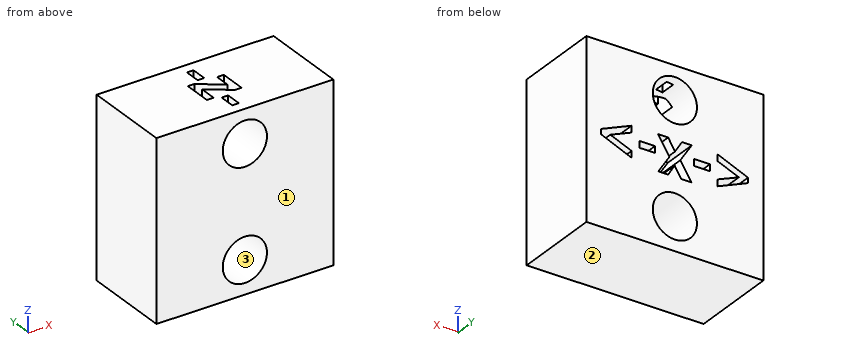
Autodesk Inventor part; units mm, degrees
ref_plane "YZ Plane" through (0, 0, 0) normal (1, 0, 0) x (0, 1, 0)
ref_plane "XZ Plane" through (0, 0, 0) normal (0, 1, 0) x (-1, 0, 0)
ref_plane "XY Plane" through (0, 0, 0) normal (0, 0, 1) x (1, 0, 0)
sketch "Sketch1" plane through (0, 0, 0) normal (0, 1, 0) x (-1, 0, 0)
  line L0 (12.7, 12.7) -> (-12.7, 12.7)
  line L1 (-12.7, 12.7) -> (-12.7, -12.7)
  line L2 (-12.7, -12.7) -> (12.7, -12.7)
  line L3 (12.7, -12.7) -> (12.7, 12.7)
  line L4 (12.7, 12.7) -> (-12.7, -12.7) construction
  line L5 (-12.7, 12.7) -> (12.7, -12.7) construction
  point P0 (0, 0)
  dimension "d0" = 25.4
  dimension "d1" = 25.4
extrude "Extrusion1" add sketch "Sketch1" along normal blind 12.7
sketch "Sketch2" plane through (0, 12.7, 0) normal (0, 1, 0) x (1, 0, 0)
  line L0 (-12.7, 12.7) -> (-12.7, -12.7) construction
  line L1 (-12.7, 0) -> (12.7, 0) construction
  line L2 (12.7, -12.7) -> (12.7, 12.7) construction
  line L3 (-6.1256, -2.4906) -> (-10.5058, -0.671)
  line L4 (-10.5058, -0.671) -> (-10.5058, 0.0782)
  line L5 (-10.5058, 0.0782) -> (-6.1256, 1.8978)
  line L6 (-6.1256, 1.8978) -> (-6.1256, 0.9551)
  line L7 (-6.1256, 0.9551) -> (-9.1885, -0.3005)
  line L8 (-9.1885, -0.3005) -> (-6.1256, -1.5479)
  line L9 (-6.1256, -1.5479) -> (-6.1256, -2.4906)
  line L10 (-2.7705, -0.7698) -> (-5.0306, -0.7698)
  line L11 (-5.0306, -0.7698) -> (-5.0306, 0.177)
  line L12 (-5.0306, 0.177) -> (-2.7705, 0.177)
  line L13 (-2.7705, 0.177) -> (-2.7705, -0.7698)
  line L14 (2.433, -2.54) -> (0.9592, -2.54)
  line L15 (0.9592, -2.54) -> (-0.0206, -0.9221)
  line L16 (-0.0206, -0.9221) -> (-1.0209, -2.54)
  line L17 (-1.0209, -2.54) -> (-2.433, -2.54)
  line L18 (-2.433, -2.54) -> (-0.7822, 0.0165)
  line L19 (-0.7822, 0.0165) -> (-2.3671, 2.54)
  line L20 (-2.3671, 2.54) -> (-0.8933, 2.54)
  line L21 (-0.8933, 2.54) -> (0.0247, 1.0045)
  line L22 (0.0247, 1.0045) -> (0.9674, 2.54)
  line L23 (0.9674, 2.54) -> (2.3794, 2.54)
  line L24 (2.3794, 2.54) -> (0.7863, 0.07)
  line L25 (0.7863, 0.07) -> (2.433, -2.54)
  line L26 (5.1088, -0.7698) -> (2.8488, -0.7698)
  line L27 (2.8488, -0.7698) -> (2.8488, 0.177)
  line L28 (2.8488, 0.177) -> (5.1088, 0.177)
  line L29 (5.1088, 0.177) -> (5.1088, -0.7698)
  line L30 (10.5881, -0.671) -> (6.208, -2.4906)
  line L31 (6.208, -2.4906) -> (6.208, -1.5479)
  line L32 (6.208, -1.5479) -> (9.2667, -0.2964)
  line L33 (9.2667, -0.2964) -> (6.208, 0.9551)
  line L34 (6.208, 0.9551) -> (6.208, 1.8978)
  line L35 (6.208, 1.8978) -> (10.5881, 0.0782)
  line L36 (10.5881, 0.0782) -> (10.5881, -0.671)
  point P0 (0, 0)
extrude "Extrusion2" cut sketch "Sketch2" against normal blind 5.08
sketch "Sketch3" plane through (-12.7, 0, 12.7) normal (0, 0, 1) x (1, 0, 0)
  line L0 (12.6794, 12.7) -> (11.6791, 12.7) construction
  line L1 (12.7, 0) -> (12.6794, 12.7) construction
  line L2 (11.9158, 8.9011) -> (11.9121, 11.1612)
  line L3 (11.9121, 11.1612) -> (12.8589, 11.1627)
  line L4 (12.8589, 11.1627) -> (12.8626, 8.9026)
  line L5 (12.8626, 8.9026) -> (11.9158, 8.9011)
  line L6 (10.153, 4.3081) -> (10.1465, 8.3342)
  line L7 (10.1465, 8.3342) -> (11.0974, 8.3358)
  line L8 (11.0974, 8.3358) -> (14.2629, 5.9985)
  line L9 (14.2629, 5.9985) -> (14.2593, 8.2174)
  line L10 (14.2593, 8.2174) -> (15.2267, 8.219)
  line L11 (15.2267, 8.219) -> (15.2328, 4.4522)
  line L12 (15.2328, 4.4522) -> (14.2654, 4.4506)
  line L13 (14.2654, 4.4506) -> (11.1164, 6.7797)
  line L14 (11.1164, 6.7797) -> (11.1204, 4.3097)
  line L15 (11.1204, 4.3097) -> (10.153, 4.3081)
  line L16 (11.9277, 1.5405) -> (11.924, 3.8005)
  line L17 (11.924, 3.8005) -> (12.8709, 3.8021)
  line L18 (12.8709, 3.8021) -> (12.8745, 1.542)
  line L19 (12.8745, 1.542) -> (11.9277, 1.5405)
extrude "Extrusion3" cut sketch "Sketch3" against normal blind 5.08
sketch "Sketch11" plane through (0, 12.7, 0) normal (0, 1, 0) x (1, 0, 0)
  circle A0 centre (0, 7.9375) radius 3.175
  circle A1 centre (0, -7.9375) radius 3.175
  line L0 (12.7, 12.7) -> (-12.7, 12.7)
  line L1 (-12.7, -12.7) -> (12.7, -12.7)
  point P0 (0, 0)
  dimension "d81" = 6.35
  dimension "d82" = 4.7625
  dimension "d83" = 4.7625
extrude "Extrusion4" cut sketch "Sketch11" against normal blind 25.4
equation "\"d46\" = 0.125 * Sketch7_Pitch"
equation "\"Sketch7_Pitch\" = 1.27"
equation "\"d48\" = 60deg"
equation "\"d67\" = 0.125 * Sketch9_Pitch"
equation "\"Sketch9_Pitch\" = 1.27"
equation "\"d69\" = 60deg"
equation "\"d99\" = 0.125 * Sketch12_Pitch"
equation "\"Sketch12_Pitch\" = 1.27"
equation "\"d101\" = 60deg"
equation "\"d120\" = 0.125 * Sketch14_Pitch"
equation "\"Sketch14_Pitch\" = 1.27"
equation "\"d122\" = 60deg"
equation "\"d143\" = 55deg"
equation "\"Sketch16_Pitch\" = 1.27"
equation "\"d161\" = 55deg"
equation "\"Sketch18_Pitch\" = 1.27"
properties part number "squareCalibrationBlock-1in"
The listing builds one solid part. Answer for the finished solid, in the listing's coordinates (mm). Face numbers are marked on the shaded views. Give positions to 0.01 mm unless a question says otherwise; leave off trailing zeros. Write each loop counter-clockwise with the first axis right and the second up, starting at its lowest first coordinate (ties: lowest second). Pieces come first, ordered by that corner, then holes.
1) For a pull along Z with two mould halves and no side action, classify the marked faces 1, 2 and 3 as pulls with the +Z half, pulls with the -Z half, needs draft (parallel to the pull), parting line crosses it, or undercut.
2) Find the intervals of material crossed by L1, parallel to Z at x = -2, y = 8; L2, parallel to Z at x = -1, y = 5.75; L3, parallel to Z at x = 0, y = 6.25, in increasing order.
3) Section A-A (z = 5.25) is taken. Write down the section's boundary in (x, y), and give its area (3 significant figures).
4) Section C-C (z = -10) is taken. Write down the section's boundary in (x, y).
5) Section D-D (y = 12.25) is taken. Count the separate pieces of the cut face and the enclosed holes in it, and give its area (3 significant figures).
6) Section B-B (x = -8) is taken. Write down the section's boundary in (y, z).
Response:
1. face 1: needs draft
1. face 2: pulls with the -Z half
1. face 3: undercut
2. L1: z = -12.7 to -10.4, -5.47 to -2.54, -1.96 to 1.87, 2.54 to 5.47
2. L2: z = -12.7 to -10.95, -4.92 to 4.92, 10.95 to 12.7
2. L3: z = -12.7 to -11.11, -4.76 to 4.76
3. outline: (-12.7, 0) - (-1.69, 0) - (-1.69, 12.7) - (-12.7, 12.7) - close; (1.69, 0) - (12.7, 0) - (12.7, 12.7) - (1.69, 12.7) - close
3. area: 280 mm2
4. outline: (-12.7, 0) - (-2.41, 0) - (-2.41, 12.7) - (-12.7, 12.7) - close; (2.41, 0) - (12.7, 0) - (12.7, 12.7) - (2.41, 12.7) - close
5. separate pieces: 1
5. enclosed holes: 7
5. area: 550 mm2
6. outline: (0, -12.7) - (12.7, -12.7) - (12.7, -1.12) - (7.62, -1.12) - (7.62, -0.19) - (12.7, -0.19) - (12.7, 0.78) - (7.62, 0.78) - (7.62, 1.71) - (12.7, 1.71) - (12.7, 12.7) - (0, 12.7) - close
